Input: part model. Units: mm. Frame: model coordinates. A direction names the side the tool comes from. Coordinates: 2 decimals unless noted, no trailing zeros. Order: outer loops, then holes, each group sorted by start corner. A loop starts at its lowest first (then second) coordinate and runs counter-clockwise, first axis right, second up. Notation, with made-up numbers: (-31.5, 20) - (-2.5, 20) arc R7 cw to (-2.5, 31) - close; hole circle Ø2 at (78.5, 40.25). An arc over 180 degrees is marked (long way). Use a Markdown table: item, result. Add a question column.
from build123d import *

# Parameters (mm, degrees)
ESQUISSE1_W             = 62
ESQUISSE1_H             = 42
BOSS_EXTRU_1_DEPTH      = 8
ESQUISSE2_R             = 2.1
ESQUISSE2_R_2           = 12.5
ESQUISSE2_R_3           = 1.7
ENL_V_MAT_EXTRU_1_DEPTH = 9
ESQUISSE3_W             = 5.8
ESQUISSE3_H             = 4
ESQUISSE3_H_2           = 6
BOSS_EXTRU_2_DEPTH      = 3
CONG_1_R                = 2
ESQUISSE4_R             = 4.5
ENL_V_MAT_EXTRU_2_DEPTH = 3


with BuildPart() as part:
    # Esquisse1 → Boss.-Extru.1 (new body)
    with BuildSketch(Plane.XY):
        Rectangle(ESQUISSE1_W, ESQUISSE1_H)
    extrude(amount=BOSS_EXTRU_1_DEPTH)

    # Esquisse2 → Enlèv. mat.-Extru.1 (cut, through all)
    with BuildSketch(Plane.XY.offset(8)):
        with Locations((21, 11)):
            Circle(ESQUISSE2_R)
        with Locations((21, -11)):
            Circle(ESQUISSE2_R)
        with Locations((-10, 0)):
            Circle(ESQUISSE2_R_2)
        with Locations((-25.5, 15.5)):
            Circle(ESQUISSE2_R_3)
        with Locations((5.5, 15.5)):
            Circle(ESQUISSE2_R_3)
        with Locations((5.5, -15.5)):
            Circle(ESQUISSE2_R_3)
        with Locations((-25.5, -15.5)):
            Circle(ESQUISSE2_R_3)
    extrude(amount=-ENL_V_MAT_EXTRU_1_DEPTH, mode=Mode.SUBTRACT)

    # Esquisse3 → Boss.-Extru.2 (add)
    with BuildSketch(Plane.XY.offset(8)):
        with Locations((21, 19)):
            Rectangle(ESQUISSE3_W, ESQUISSE3_H)
        with Locations((21, -19)):
            Rectangle(ESQUISSE3_W, ESQUISSE3_H)
        with Locations((21, 0)):
            Rectangle(ESQUISSE3_W, ESQUISSE3_H_2)
    extrude(amount=BOSS_EXTRU_2_DEPTH)

    # Congé1
    cong_1_edges = [part.edges().sort_by_distance(p)[0] for p in [
        (-31, 21, 4),
        (-31, -21, 4),
        (31, 21, 4),
        (31, -21, 4),
    ]]
    fillet(cong_1_edges, radius=CONG_1_R)

    # Esquisse4 → Enlèv. mat.-Extru.2 (cut)
    with BuildSketch(Plane.XY.offset(8)):
        with Locations((-25.5, 15.5)):
            Circle(ESQUISSE4_R)
        with Locations((-25.5, -15.5)):
            Circle(ESQUISSE4_R)
        with Locations((5.5, -15.5)):
            Circle(ESQUISSE4_R)
        with Locations((5.5, 15.5)):
            Circle(ESQUISSE4_R)
    extrude(amount=-ENL_V_MAT_EXTRU_2_DEPTH, mode=Mode.SUBTRACT)


solid = part.part
1) Cut plane C-C (y = 0). Return the cut outline in (x, z).
2) Pull-direction query (X, two-part tool) for faces 5 (the flat face through (21, -3, 9)), 6 (the flat face through (31, 0, 4)), 7 (the cylindrical face through (7.919, 19.294, 6.521)); classes: pulls with the +X half, pulls with the -X half, needs draft (parallel to the pull), parting line crosses it, or undercut.
3) Reachability of faces 1 (the cylindrical face through (-28.82, -12.46, 6.52)), 2 (the flat face through (21, -17, 9)), 3 (the flat face through (18.1, -19, 9)), 4 (the flat face through (23.9, -19, 9)) from +Z, -Z, +X, -X, +Y, -Y: full face, straight path, thin tool, end or side. Return the list, or none.
4) Cut plane D-D (z = 2). Return the cut outline in (x, y), and give its area (3 significant figures).
5) Contact query for flat-ended pins moving along their axis: P1, Ø5, axis at y = 2.5, z = 8.5, coming from the +X side; P2, Ø0.9, axis at y = 19.5, z = 9.5, coming from the -X side; P3, Ø5, axis at x = 18, y = 6, coming from the +Z side; P4, Ø2.5, axis at x = 4, y = 15, coming from the +Z side. Output: stop coordinate, or through.
6) Cut plane B-B (z = 9.5). Return the cut outline in (x, y).
7) Cut plane A-A (x = -10). Return the cut outline in (y, z), and give its area (3 significant figures).
8) Material intervals for L1, parallel to Y at x = 21, z = 3.5; L2, parallel to Y at x = -25.5, z = 6.85; L3, parallel to Y at x = -9.5, z = 1, sorted ascending.
Computed:
| question | item | result |
|---|---|---|
| 1 | outline | (-31, 0) - (-22.5, 0) - (-22.5, 8) - (-31, 8) - close; (2.5, 0) - (31, 0) - (31, 8) - (23.9, 8) - (23.9, 11) - (18.1, 11) - (18.1, 8) - (2.5, 8) - close |
| 2 | face 5 | needs draft |
| 2 | face 6 | pulls with the +X half |
| 2 | face 7 | undercut |
| 3 | face 1 | +Z |
| 3 | face 2 | +Z, +X, -X |
| 3 | face 3 | +Z, -X, +Y, -Y |
| 3 | face 4 | +Z, +X, +Y, -Y |
| 4 | outline | (-31, -19) arc R2 ccw to (-29, -21) - (29, -21) arc R2 ccw to (31, -19) - (31, 19) arc R2 ccw to (29, 21) - (-29, 21) arc R2 ccw to (-31, 19) - close; hole circle Ø3.4 at (-25.5, -15.5); hole circle Ø3.4 at (-25.5, 15.5); hole circle Ø25 at (-10, 0); hole circle Ø3.4 at (5.5, -15.5); hole circle Ø3.4 at (5.5, 15.5); hole circle Ø4.2 at (21, -11); hole circle Ø4.2 at (21, 11) |
| 4 | area | 2,050 mm2 |
| 5 | P1 | stops at x = 31 |
| 5 | P2 | stops at x = 18.1 |
| 5 | P3 | stops at z = 8 |
| 5 | P4 | stops at z = 5 |
| 6 | outline | (18.1, -21) - (23.9, -21) - (23.9, -17) - (18.1, -17) - close; (18.1, -3) - (23.9, -3) - (23.9, 3) - (18.1, 3) - close; (18.1, 17) - (23.9, 17) - (23.9, 21) - (18.1, 21) - close |
| 7 | outline | (-21, 0) - (-12.5, 0) - (-12.5, 8) - (-21, 8) - close; (12.5, 0) - (21, 0) - (21, 8) - (12.5, 8) - close |
| 7 | area | 136 mm2 |
| 8 | L1 | y = -21 to -13.1, -8.9 to 8.9, 13.1 to 21 |
| 8 | L2 | y = -21 to -20, -11 to 11, 20 to 21 |
| 8 | L3 | y = -21 to -12.49, 12.49 to 21 |
